Work out the finished part from the listing and answer in its coordinate system (mm). A direction names the side the tool comes from. Coordinates: 2 decimals unless noted, no trailing zeros. Write each loop counter-clockwise with the first axis right and the second up, starting at its lowest first coordinate (ties: lowest second). Pieces come first, ordered by that corner, then holes. Notation, with made-up numbers: (81, 76) - (135, 76) arc R24 ccw to (135, 110) - close; hole circle Ø4 at (36, 10.5). An arc over 180 degrees is marked (long way). One line per item, written item: value.
```python
from build123d import *

# Parameters (mm, degrees)
SKETCH5_W            = 450
SKETCH5_H            = 350
BOSS_EXTRUDE1_DEPTH  = 2
FILLET1_R            = 10
CUT_EXTRUDE1_DEPTH   = 571.091220771
M4_CLEARANCE_HOLE1_D = 4.5
SKETCH13_R           = 1.75
CUT_EXTRUDE2_DEPTH   = 571.091220771
SKETCH14_R           = 1.75
CUT_EXTRUDE3_DEPTH   = 571.091220771
SKETCH15_W           = 125
SKETCH15_H           = 50
CUT_EXTRUDE4_DEPTH   = 571.091220771
FILLET2_R            = 10
SKETCH16_R           = 1.65
CUT_EXTRUDE5_DEPTH   = 571.091220771


with BuildPart() as part:
    # Sketch5 → Boss-Extrude1 (new body)
    with BuildSketch(Plane(origin=(0, 0, 0), x_dir=(1, 0, 0), z_dir=(0, 1, 0))):
        with Locations((225, 175)):
            Rectangle(SKETCH5_W, SKETCH5_H)
    extrude(amount=BOSS_EXTRUDE1_DEPTH)

    # Fillet1
    fillet1_edges = [part.edges().sort_by_distance(p)[0] for p in [
        (0, 1, 0),
        (0, 1, -350),
        (450, 1, -350),
        (450, 1, 0),
    ]]
    fillet(fillet1_edges, radius=FILLET1_R)

    # Sketch6 → Cut-Extrude1 (cut, through all)
    with BuildSketch(Plane(origin=(0, 2, 0), x_dir=(1, 0, 0), z_dir=(0, 1, 0))):
        with BuildLine():
            Line((140, 190), (140, 160))
            ThreePointArc((140, 160), (137.071067812, 152.928932188), (130, 150))
            Line((130, 150), (60, 150))
            ThreePointArc((60, 150), (52.928932188, 152.928932188), (50, 160))
            Line((50, 160), (50, 190))
            ThreePointArc((50, 190), (52.928932188, 197.071067812), (60, 200))
            Line((60, 200), (130, 200))
            ThreePointArc((130, 200), (137.071067812, 197.071067812), (140, 190))
        make_face()
    extrude(amount=-CUT_EXTRUDE1_DEPTH, mode=Mode.SUBTRACT)

    # M4 Clearance Hole1 (through all)
    with Locations(Plane(origin=(0, 2, 0), x_dir=(1, 0, 0), z_dir=(0, 1, 0))):
        with Locations((135, 10), (135, 30), (10, 90), (30, 90), (315, 10), (315, 30), (420, 90), (440, 90), (440, 260), (420, 260), (315, 340), (315, 320), (135, 340), (135, 320), (30, 260), (10, 260)):
            Hole(M4_CLEARANCE_HOLE1_D / 2)

    # Sketch13 → Cut-Extrude2 (cut, through all)
    with BuildSketch(Plane(origin=(0, 2, 0), x_dir=(1, 0, 0), z_dir=(0, 1, 0))):
        with Locations(Location((272.499999169, 35.5, 0), (0, 0, 90))):
            Circle(SKETCH13_R)
        with Locations(Location((272.499999169, 10.5, 0), (0, 0, 90))):
            Circle(SKETCH13_R)
        with Locations(Location((177.499999169, 35.5, 0), (0, 0, 90))):
            Circle(SKETCH13_R)
        with Locations(Location((177.499999169, 10.5, 0), (0, 0, 90))):
            Circle(SKETCH13_R)
        with Locations(Location((35, 222.5, 0), (0, 0, 270))):
            Circle(SKETCH13_R)
        with Locations(Location((60, 222.5, 0), (0, 0, 270))):
            Circle(SKETCH13_R)
        with Locations(Location((60, 127.5, 0), (0, 0, 270))):
            Circle(SKETCH13_R)
        with Locations(Location((35, 127.5, 0), (0, 0, 270))):
            Circle(SKETCH13_R)
        with Locations(Location((177.499999169, 339.5, 0), (0, 0, 270))):
            Circle(SKETCH13_R)
        with Locations(Location((272.499999169, 339.5, 0), (0, 0, 270))):
            Circle(SKETCH13_R)
        with Locations(Location((272.499999169, 314.5, 0), (0, 0, 270))):
            Circle(SKETCH13_R)
        with Locations(Location((177.499999169, 314.5, 0), (0, 0, 270))):
            Circle(SKETCH13_R)
        with Locations(Location((415, 127.5, 0), (0, 0, 90))):
            Circle(SKETCH13_R)
        with Locations(Location((390, 127.5, 0), (0, 0, 90))):
            Circle(SKETCH13_R)
        with Locations(Location((390, 222.5, 0), (0, 0, 90))):
            Circle(SKETCH13_R)
        with Locations(Location((415, 222.5, 0), (0, 0, 90))):
            Circle(SKETCH13_R)
    extrude(amount=-CUT_EXTRUDE2_DEPTH, mode=Mode.SUBTRACT)

    # Sketch14 → Cut-Extrude3 (cut, through all)
    with BuildSketch(Plane(origin=(0, 2, 0), x_dir=(1, 0, 0), z_dir=(0, 1, 0))):
        with Locations(Location((27.5, 76.9004, 0), (0, 0, 270))):
            Circle(SKETCH14_R)
        with Locations(Location((67.5, 76.9004, 0), (0, 0, 270))):
            Circle(SKETCH14_R)
        with Locations(Location((67.5, 66.9004, 0), (0, 0, 270))):
            Circle(SKETCH14_R)
        with Locations(Location((27.5, 66.9004, 0), (0, 0, 270))):
            Circle(SKETCH14_R)
        with Locations(Location((67.5, 283.0996, 0), (0, 0, 90))):
            Circle(SKETCH14_R)
        with Locations(Location((67.5, 273.0996, 0), (0, 0, 90))):
            Circle(SKETCH14_R)
        with Locations(Location((27.5, 283.0996, 0), (0, 0, 90))):
            Circle(SKETCH14_R)
        with Locations(Location((27.5, 273.0996, 0), (0, 0, 90))):
            Circle(SKETCH14_R)
        with Locations(Location((382.5, 273.0996, 0), (0, 0, 270))):
            Circle(SKETCH14_R)
        with Locations(Location((382.5, 283.0996, 0), (0, 0, 270))):
            Circle(SKETCH14_R)
        with Locations(Location((422.5, 283.0996, 0), (0, 0, 270))):
            Circle(SKETCH14_R)
        with Locations(Location((422.5, 273.0996, 0), (0, 0, 270))):
            Circle(SKETCH14_R)
        with Locations(Location((422.5, 66.9004, 0), (0, 0, 90))):
            Circle(SKETCH14_R)
        with Locations(Location((382.5, 66.9004, 0), (0, 0, 90))):
            Circle(SKETCH14_R)
        with Locations(Location((382.5, 76.9004, 0), (0, 0, 90))):
            Circle(SKETCH14_R)
        with Locations(Location((422.5, 76.9004, 0), (0, 0, 90))):
            Circle(SKETCH14_R)
    extrude(amount=-CUT_EXTRUDE3_DEPTH, mode=Mode.SUBTRACT)

    # Sketch15 → Cut-Extrude4 (cut, through all)
    with BuildSketch(Plane(origin=(0, 2, 0), x_dir=(1, 0, 0), z_dir=(0, 1, 0))):
        with Locations((62.5, 325)):
            Rectangle(SKETCH15_W, SKETCH15_H)
        with Locations((62.5, 25)):
            Rectangle(SKETCH15_W, SKETCH15_H)
        with Locations((387.5, 25)):
            Rectangle(SKETCH15_W, SKETCH15_H)
        with Locations((387.5, 325)):
            Rectangle(SKETCH15_W, SKETCH15_H)
    extrude(amount=-CUT_EXTRUDE4_DEPTH, mode=Mode.SUBTRACT)

    # Fillet2
    fillet2_edges = [part.edges().sort_by_distance(p)[0] for p in [
        (325, 1, -350),
        (450, 1, -300),
        (450, 1, -50),
        (325, 1, 0),
        (125, 1, 0),
        (0, 1, -50),
        (0, 1, -300),
        (125, 1, -350),
    ]]
    fillet(fillet2_edges, radius=FILLET2_R)

    # Sketch16 → Cut-Extrude5 (cut, through all)
    with BuildSketch(Plane(origin=(0, 2, 0), x_dir=(1, 0, 0), z_dir=(0, 1, 0))):
        with Locations(Location((39, 197.3, 0), (0, 0, 270))):
            Circle(SKETCH16_R)
        with Locations(Location((39, 152.7, 0), (0, 0, 270))):
            Circle(SKETCH16_R)
        with Locations(Location((151, 152.7, 0), (0, 0, 90))):
            Circle(SKETCH16_R)
        with Locations(Location((151, 197.3, 0), (0, 0, 90))):
            Circle(SKETCH16_R)
    extrude(amount=-CUT_EXTRUDE5_DEPTH, mode=Mode.SUBTRACT)


solid = part.part
```
Item 1: Section C-C, the plane y = 0.4 is taken. Give the number of separate pieces and of enclosed holes in the cut face, then the cut area to 3 significant figures.
Evaluation:
separate pieces: 1
enclosed holes: 53
area: 127,000 mm2
Item 2: Which of the six approach directions +Z, -Z, +X, -X, +Y, -Y give full straight-line access (tool end or side, diameter ignored) to faces 1 (the face through (136.99, 1.01, -197.15)), 2 (the face through (128.01, 0.99, -2.85))?
Evaluation:
face 1: +Y, -Y
face 2: +Z, -X, +Y, -Y
Item 3: Section D-D, the plane x = 340.5 is taken. Determine the outline of the cut face in (y, z).
Evaluation:
outline: (0, -300) - (2, -300) - (2, -50) - (0, -50) - close
Item 4: Section B-B, the plane z = -42 is taken. Determine the outline of the cut face in (x, y), then the cut area to 3 significant figures.
Evaluation:
outline: (125, 0) - (325, 0) - (325, 2) - (125, 2) - close
area: 400 mm2
Item 5: Section A-A, the plane x = 107.5 is taken. Determine the outline of the cut face in (y, z), then the cut area to 3 significant figures.
Evaluation:
outline: (0, -300) - (2, -300) - (2, -200) - (0, -200) - close; (0, -150) - (2, -150) - (2, -50) - (0, -50) - close
area: 400 mm2
Item 6: Determine the mould class of faces 3 (the face through (137.15, 1.01, -153.01)), 4 (the face through (447.15, 0.99, -53.01)), 5 (the face through (2.85, 0.99, -296.99)) for opening direction X: +X half, -X half, draft (parallel to the pull), parting line (faces both ways), or undercut.
Evaluation:
face 3: undercut
face 4: +X half
face 5: -X half
Item 7: Given pin 1 (0.6 mm diameter, centred on x = 47, y = 1, fed in from +Z), flat-ended and moving along its own axis, determine where the tip first touches the part or whether it passes through.
Evaluation:
pin 1: stops at z = -50
Item 8: Consider probe 1 along X at (y, z) = (1.3, -320); probe 2 along X at (y, z) = (0.9, -260); probe 3 along Z at (x, y) = (315, 1.25). Determine where each line is inside the solid, lowest interval first.
Evaluation:
probe 1: x = 125 to 132.75, 137.25 to 312.75, 317.25 to 325
probe 2: x = 0 to 7.75, 12.25 to 27.75, 32.25 to 417.75, 422.25 to 437.75, 442.25 to 450
probe 3: z = -350 to -342.25, -337.75 to -322.25, -317.75 to -32.25, -27.75 to -12.25, -7.75 to 0
